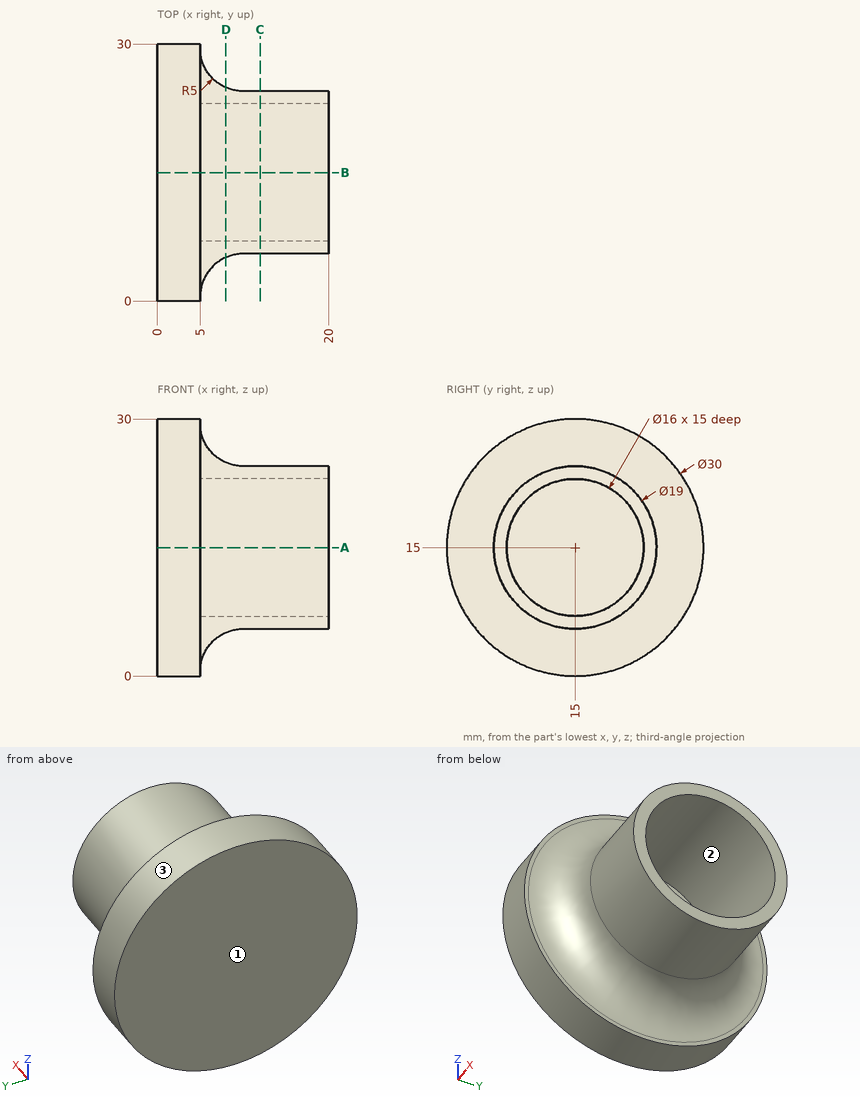
Job drawing, mm, ordinate dimensions from the low corner. One solid piece. Coordinates: 2 decimals unless noted, no trailing zeros. Order: outer loops, then holes, each group sorted by start corner. A loop starts at its lowest first (then second) coordinate and runs counter-clockwise, first axis right, second up. Notation, with made-up numbers: (25, 80) -> (51, 80) arc R12 cw to (51, 90) -> close; hole circle Ø3 at (-7.75, 11). An arc over 180 degrees is marked (long way). Return JSON: item names as keys, results as strings. Group by question number.
Item 1: Pull direction Y, two halves, no side cores. Call the marked faces 1, 2 and 3: pulls with the +Y half, pulls with the -Y half, needs draft (parallel to the pull), parting line crosses it, or undercut.
Item 2: Flat gauge pins, fed straight in: P1, Ø4, axis at x = 13, z = 19, coming from the +Y side; P2, Ø6, axis at x = 6.5, z = 20, coming from the +Y side; P3, Ø5, axis at y = 13, z = 12, coming from the +X side. Where does each tip first touch, or does it go through?
Item 3: Saw through at A-A on z = 15. Write the cut outline in (x, y), then the cut area to 3 significant figures.
Item 4: Wall check: line 1 along Y through (x, z) = (14.5, 15); line 2 along X through (y, z) = (15.75, 13). Give the ranges that are in metal, low to high. Write a range as [from, to].
Item 5: Saw through at C-C on x = 12. Write the cut outline in (y, z).
Item 6: Saw through at D-D on x = 8. Write the cut outline in (y, z), then the cut area to 3 significant figures.
Values found:
{
 "1": {"face 1": "needs draft", "face 2": "undercut", "face 3": "parting line crosses it"},
 "2": {"P1": "stops at y = 24.29", "P2": "stops at y = 29.81", "P3": "stops at x = 5"},
 "3": {"outline": "(0, 0) -> (5, 0) -> (5, 0.5) arc R5 cw to (10, 5.5) -> (20, 5.5) -> (20, 7) -> (5, 7) -> (5, 23) -> (20, 23) -> (20, 24.5) -> (10, 24.5) arc R5 cw to (5, 29.5) -> (5, 30) -> (0, 30) -> close", "area": "206 mm2"},
 "4": {"line 1": "y = [5.5, 7], [23, 24.5]", "line 2": "x = [0, 5]"},
 "5": {"outline": "circle Ø19 at (15, 15); hole circle Ø16 at (15, 15)"},
 "6": {"outline": "circle Ø19.83 at (15, 15); hole circle Ø16 at (15, 15)", "area": "108 mm2"}
}
